```python
from build123d import *

# Parameters (mm, degrees)
BOSS_EXTRUDE1_DEPTH      = 10
FILLET1_R                = 10
FILLET2_R                = 5
BOSS_EXTRUDE2_DEPTH      = 10
BOSS_EXTRUDE2_DEPTH_BACK = 40
SKETCH2_R                = 7
BOSS_EXTRUDE3_START      = -5
SKETCH3_R                = 5
BOSS_EXTRUDE3_DEPTH      = 15
CHAMFER1_SIZE            = 2.5
BOSS_EXTRUDE4_DEPTH      = 18
BOSS_EXTRUDE4_DEPTH_BACK = 10
SKETCH4_R                = 13
SKETCH5_R                = 13.358898944
BOSS_EXTRUDE5_DEPTH      = 4


with BuildPart() as part:
    # Sketch1 → Boss-Extrude1 (new body)
    with BuildSketch(Plane.XY):
        Polygon((-58.818184361, 21.563458262), (11.382033939, 21.563458262), (11.382033939, 7.563458262), (-34.282866194, -6.436541738), (-58.818184361, -6.436541738), align=None)
    extrude(amount=BOSS_EXTRUDE1_DEPTH)

    # Fillet1
    fillet1_edges = [part.edges().sort_by_distance(p)[0] for p in [
        (-58.818184361, 21.563458262, 5),
        (-58.818184361, -6.436541738, 5),
    ]]
    fillet(fillet1_edges, radius=FILLET1_R)

    # Fillet2
    fillet2_edges = [part.edges().sort_by_distance(p)[0] for p in [
        (11.382033939, 21.563458262, 5),
        (11.382033939, 7.563458262, 5),
        (-34.282866194, -6.436541738, 5),
    ]]
    fillet(fillet2_edges, radius=FILLET2_R)

    # Sketch2 → Boss-Extrude2 (add, two sides: drawn at the far end of the back side and taken through both)
    with BuildSketch(Plane(origin=(0, 21.563458262, 0), x_dir=(1, 0, 0), z_dir=(0, 1, 0)).offset(-BOSS_EXTRUDE2_DEPTH_BACK)):
        with Locations(Location((-48.818184361, -5, 0), (0, 0, 270))):
            Circle(SKETCH2_R)
    extrude(amount=BOSS_EXTRUDE2_DEPTH + BOSS_EXTRUDE2_DEPTH_BACK)

    # Sketch3 → Boss-Extrude3 (add)
    with BuildSketch(Plane(origin=(0, 21.563458262, 0), x_dir=(1, 0, 0), z_dir=(0, 1, 0)).offset(BOSS_EXTRUDE3_START)):
        with Locations(Location((6.382033939, -5, 0), (0, 0, 270))):
            Circle(SKETCH3_R)
    extrude(amount=BOSS_EXTRUDE3_DEPTH)

    # Chamfer1
    chamfer1_edges = [part.edges().sort_by_distance(p)[0] for p in [
        (-48.818184361, -18.436541738, -2),
        (-48.818184361, 31.563458262, -2),
        (6.382033939, 31.563458262, 0),
    ]]
    chamfer(chamfer1_edges, length=CHAMFER1_SIZE)

    # Sketch4 → Boss-Extrude4 (add, two sides: drawn at the far end of the back side and taken through both)
    with BuildSketch(Plane(origin=(0, 0, 0), x_dir=(-1, 0, 0), z_dir=(0, 0, -1)).offset(-BOSS_EXTRUDE4_DEPTH_BACK)):
        with Locations((43.919204876, 8.204559319)):
            Circle(SKETCH4_R)
    extrude(amount=BOSS_EXTRUDE4_DEPTH + BOSS_EXTRUDE4_DEPTH_BACK)

    # Sketch5 → Boss-Extrude5 (add)
    with BuildSketch(Plane(origin=(0, 0, 0), x_dir=(-1, 0, 0), z_dir=(0, 0, -1))):
        with Locations(Location((43.919204876, 8.204559319, 0), (0, 0, 90))):
            Circle(SKETCH5_R)
    extrude(amount=BOSS_EXTRUDE5_DEPTH)


solid = part.part
```
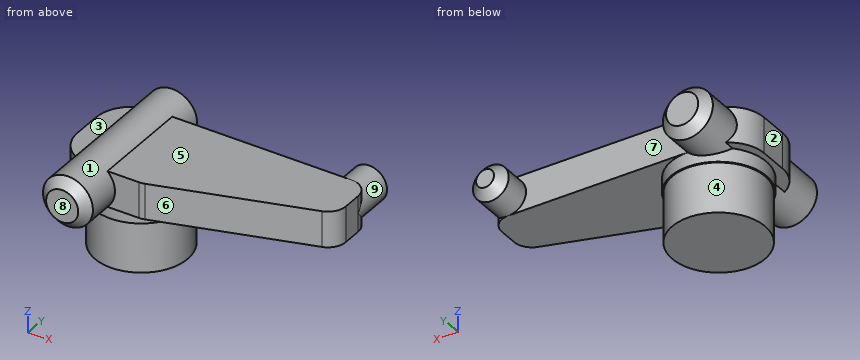
Part model, mm, in its own coordinate system. Face numbers are marked on the shaded views. A direction names the side the tool comes from. Round coordinates to 2 decimals unless told otherwise and drop trailing zeros. Loops run counter-clockwise (first coordinate to the right, second up) from the corner with the lowest first, then second, coordinate; pieces in that order, holes last.
Item 1: Cut at C-C, the plane z = -6.5. Give the cut face in (x, y).
Item 2: Cut at D-D, the plane x = -18. Give the cut face in (y, z), then the cut area to 3 significant figures.
Item 3: 3-axis set-ups, long thin cutter, end or side, ignore diameter. For the marked faces 1, 2, 3, 4 and 5: which of +Z, -Z, +X, -X, +Y, -Y reach the whole face in a straight line?
Item 4: Cut at A-A, the plane x = -32.5. Give the cut face in (y, z), then the cut area to 3 significant figures.
Item 5: Mould opens along X. For the marked faces 6, 7, 8 and 9 say: +X half, -X half, draft (parallel to the pull), parting line (faces both ways), or undercut.
Item 6: Cut at B-B, the plane y = 13.5. Give the cut face in (x, z).
Item 7: Drop flat-ended pins along their axis: P1, Ø1, axis at x = -23, y = 21.5, coming from the -Z side; P2, Ø5, axis at x = -7, z = 4.5, coming from the +Y side; P3, Ø1, axis at y = 7, z = -9, coming from the -X side; P4, Ø10, axis at y = -10.5, z = -15, coming from the +X side. Give the stop position or say it passes through.
Item 8: Drill centre lines: line 1 (Z direction, x = 7.5, y = 19.5); line 2 (Z direction, x = -39, y = 13); line 3 (X direction, y = 11, z = 9). Where is each one in solid material? Low to high.
A:
1. outline: circle Ø26 at (-43.92, 8.2)
2. outline: (-1.44, 0) - (21.56, 0) - (21.56, 10) - (-1.44, 10) - close
2. area: 230 mm2
3. face 1: none
3. face 2: +Z, -Z, -X, +Y, -Y
3. face 3: +Z, -X, +Y, -Y
3. face 4: -Z
3. face 5: +Z, +X, +Y, -Y
4. outline: (-5.89, 0) - (1.27, 0) - (1.27, -4) - (1.99, -4) - (1.99, -18) - (14.42, -18) - (14.42, -4) - (15.14, -4) - (15.14, 0) - (21.56, 0) - (21.56, 10) - (-5.89, 10) - close
4. area: 504 mm2
5. face 6: +X half
5. face 7: undercut
5. face 8: draft
5. face 9: undercut
6. outline: (-58.63, 0) - (-56.18, 0) - (-56.18, -4) - (-55.79, -4) - (-55.79, -18) - (-32.05, -18) - (-32.05, -4) - (-31.65, -4) - (-31.65, 0) - (11.38, 0) - (11.38, 10) - (-43.92, 10) arc R7 ccw to (-53.72, 10) - (-58.63, 10) - close
7. P1: stops at z = 0
7. P2: stops at y = 21.56
7. P3: stops at x = -56.9
7. P4: passes through
8. line 1: z = 0 to 10
8. line 2: z = -18 to 10
8. line 3: x = -58.82 to 11.38
